```python
from build123d import *

# Parameters (mm, degrees)
F0_R     = 2.5
F1_DEPTH = 7
F2_R     = 2.75
F3_DEPTH = 1
F4_R     = 2.75
F5_DEPTH = 1


with BuildPart() as f1:
    # F0 (on Front) → F1 (new body)
    with BuildSketch(Plane.XZ):
        with BuildLine():
            ThreePointArc((35, -3.5), (38.5, 0), (35, 3.5))
            Line((35, 3.5), (-35, 3.5))
            ThreePointArc((-35, 3.5), (-38.5, 0), (-35, -3.5))
            Line((-35, -3.5), (35, -3.5))
        make_face()
        with Locations((-35, 0)):
            Circle(F0_R, mode=Mode.SUBTRACT)
        with Locations((-26.25, 0)):
            Circle(F0_R, mode=Mode.SUBTRACT)
        with Locations((-17.5, 0)):
            Circle(F0_R, mode=Mode.SUBTRACT)
        with Locations((-8.75, 0)):
            Circle(F0_R, mode=Mode.SUBTRACT)
        with Locations((0, 0)):
            Circle(F0_R, mode=Mode.SUBTRACT)
        with Locations((8.75, 0)):
            Circle(F0_R, mode=Mode.SUBTRACT)
        with Locations((17.5, 0)):
            Circle(F0_R, mode=Mode.SUBTRACT)
        with Locations((26.25, 0)):
            Circle(F0_R, mode=Mode.SUBTRACT)
        with Locations((35, 0)):
            Circle(F0_R, mode=Mode.SUBTRACT)
    extrude(amount=F1_DEPTH)

    # F2 (on face) → F3 (cut)
    with BuildSketch(Plane(origin=(0, 0, 0), x_dir=(-1, 0, 0), z_dir=(0, 1, 0))):
        with Locations((35, 0)):
            Circle(F2_R)
        with Locations((26.25, 0)):
            Circle(F2_R)
        with Locations((17.5, 0)):
            Circle(F2_R)
        with Locations((8.75, 0)):
            Circle(F2_R)
        with Locations((0, 0)):
            Circle(F2_R)
        with Locations((-8.75, 0)):
            Circle(F2_R)
        with Locations((-17.5, 0)):
            Circle(F2_R)
        with Locations((-26.25, 0)):
            Circle(F2_R)
        with Locations((-35, 0)):
            Circle(F2_R)
    extrude(amount=-F3_DEPTH, mode=Mode.SUBTRACT)

    # F4 (on face) → F5 (cut)
    with BuildSketch(Plane.XZ.offset(7)):
        with Locations((-35, 0)):
            Circle(F4_R)
        with Locations((-26.25, 0)):
            Circle(F4_R)
        with Locations((-17.5, 0)):
            Circle(F4_R)
        with Locations((-8.75, 0)):
            Circle(F4_R)
        with Locations((0, 0)):
            Circle(F4_R)
        with Locations((8.75, 0)):
            Circle(F4_R)
        with Locations((17.5, 0)):
            Circle(F4_R)
        with Locations((26.25, 0)):
            Circle(F4_R)
        with Locations((35, 0)):
            Circle(F4_R)
    extrude(amount=-F5_DEPTH, mode=Mode.SUBTRACT)


solid = f1.part
```
Could you check a few things on this model? Use its own coordinates, in mm. A direction names the side the tool comes from. Coordinates: 2 decimals unless noted, no trailing zeros. Loops run counter-clockwise (first coordinate to the right, second up) from the corner with the lowest first, then second, coordinate; pieces in that order, holes last. Notation, with made-up numbers: M 50.5,20.5 L 75.5,20.5 A20 cw 75.5,25.5 Z; hole C 4,29.5 d5. An arc over 180 degrees is marked long. Put each result on its own line as item: value. Start each with the question number.
(1) For faces 1 (the face through (23.752, -3.465, 0.11)), 2 (the face through (32.253, -6.507, 0.121)), 3 (the face through (37.747, -0.493, 0.121)), which set-ups out of +Z, -Z, +X, -X, +Y, -Y let a thin tool reach every point of the face, with its end or its side?
(2) Suppose I cut it at A-A on y = -3.25. Count the separate pieces of the cut face and the enclosed holes in it, then the cut area to 3 significant figures.
(3) I need wall thicknesses on line 1 (Z direction, x = -35, y = -0.25); line 2 (Z direction, x = -26, y = -1.75); line 3 (X direction, y = -2.5, z = 2.75). Which ranges of each line are inside material? Lowest first, please. Write a range as from..to.
(4) Suppose I cut it at D-D on x = -27. Please give me the cut outline in (y, z), then the cut area to 3 significant figures.
(5) Suppose I cut it at B-B on x = -8.75. Please give me the cut outline in (y, z).
(6) Will these pins go through, and if not, where does the flat tip stop? P1, Ø4, axis at y = -4.5, z = -2.5, coming from the +X side; P2, Ø1, axis at y = -3.5, z = 1.5, coming from the -X side; P3, Ø1.6, axis at x = -27.5, z = -1, coming from the -Y side; P4, Ø1, axis at y = -3.5, z = -1.5, coming from the +X side.
(7) Thinking about a two-plate mould opening in Z: for faces 4 (the face through (-11.248, -3.465, 0.11)), 5 (the face through (0, -3, -3.5)), 6 (the face through (-3, -7, 1)), which applies, pulls with the +Z half, pulls with the -Z half, needs draft (parallel to the pull), parting line crosses it, or undercut?
Solutions:
1. face 1: +Y, -Y
1. face 2: -Y
1. face 3: +Y
2. separate pieces: 1
2. enclosed holes: 9
2. area: 352 mm2
3. line 1: z = -3.5..-2.75, 2.75..3.5
3. line 2: z = -3.5..-2.49, 2.49..3.5
3. line 3: x = -37.17..37.17
4. outline: M -7,-3.5 L 0,-3.5 L 0,-2.65 L -1,-2.65 L -1,-2.38 L -6,-2.38 L -6,-2.65 L -7,-2.65 Z; M -7,2.65 L -6,2.65 L -6,2.38 L -1,2.38 L -1,2.65 L 0,2.65 L 0,3.5 L -7,3.5 Z
4. area: 14.6 mm2
5. outline: M -7,-3.5 L 0,-3.5 L 0,-2.75 L -1,-2.75 L -1,-2.5 L -6,-2.5 L -6,-2.75 L -7,-2.75 Z; M -7,2.75 L -6,2.75 L -6,2.5 L -1,2.5 L -1,2.75 L 0,2.75 L 0,3.5 L -7,3.5 Z
6. P1: stops at x = 38.46
6. P2: stops at x = -38.35
6. P3: passes through
6. P4: stops at x = 38.35
7. face 4: undercut
7. face 5: pulls with the -Z half
7. face 6: needs draft
